from build123d import *

# Parameters (mm, degrees)
F0_R     = 4
F0_R_2   = 22.606
F1_DEPTH = 18


with BuildPart() as f1:
    # F0 (on Front) → F1 (new body)
    with BuildSketch(Plane.XZ):
        with BuildLine():
            ThreePointArc((138.72574, -5.657885), (138.812234, -2.82953), (138.841069, 0))
            ThreePointArc((138.841069, 0), (138.546757, 9.035416), (137.665067, 18.032525))
            ThreePointArc((137.665067, 18.032525), (136.023008, 27.831344), (133.684401, 37.487643))
            ThreePointArc((133.684401, 37.487643), (129.994558, 48.76738), (125.354902, 59.690796))
            ThreePointArc((125.354902, 59.690796), (120.76521, 68.502602), (115.557102, 76.963619))
            ThreePointArc((115.557102, 76.963619), (108.562222, 86.551062), (100.774126, 95.506115))
            ThreePointArc((100.774126, 95.506115), (93.686072, 102.468348), (86.118269, 108.90586))
            ThreePointArc((86.118269, 108.90586), (76.50306, 115.862524), (66.328876, 121.972631))
            ThreePointArc((66.328876, 121.972631), (57.436288, 126.403779), (48.249579, 130.187636))
            ThreePointArc((48.249579, 130.187636), (36.955245, 133.832554), (25.390894, 136.499615))
            ThreePointArc((25.390894, 136.499615), (15.56424, 137.965927), (5.657885, 138.72574))
            ThreePointArc((5.657885, 138.72574), (-6.210007, 138.702121), (-18.032525, 137.665067))
            ThreePointArc((-18.032525, 137.665067), (-27.831344, 136.023008), (-37.487643, 133.684401))
            ThreePointArc((-37.487643, 133.684401), (-48.76738, 129.994558), (-59.690796, 125.354902))
            ThreePointArc((-59.690796, 125.354902), (-68.502602, 120.76521), (-76.963619, 115.557102))
            ThreePointArc((-76.963619, 115.557102), (-86.551062, 108.562222), (-95.506115, 100.774126))
            ThreePointArc((-95.506115, 100.774126), (-102.468348, 93.686072), (-108.90586, 86.118269))
            ThreePointArc((-108.90586, 86.118269), (-115.862524, 76.50306), (-121.972631, 66.328876))
            ThreePointArc((-121.972631, 66.328876), (-126.403779, 57.436288), (-130.187636, 48.249579))
            ThreePointArc((-130.187636, 48.249579), (-133.832554, 36.955245), (-136.499615, 25.390894))
            ThreePointArc((-136.499615, 25.390894), (-137.965927, 15.56424), (-138.72574, 5.657885))
            ThreePointArc((-138.72574, 5.657885), (-138.702121, -6.210007), (-137.665067, -18.032525))
            ThreePointArc((-137.665067, -18.032525), (-136.023008, -27.831344), (-133.684401, -37.487643))
            ThreePointArc((-133.684401, -37.487643), (-129.994558, -48.76738), (-125.354902, -59.690796))
            ThreePointArc((-125.354902, -59.690796), (-120.76521, -68.502602), (-115.557102, -76.963619))
            ThreePointArc((-115.557102, -76.963619), (-108.562222, -86.551062), (-100.774126, -95.506115))
            ThreePointArc((-100.774126, -95.506115), (-93.686072, -102.468348), (-86.118269, -108.90586))
            ThreePointArc((-86.118269, -108.90586), (-76.50306, -115.862524), (-66.328876, -121.972631))
            ThreePointArc((-66.328876, -121.972631), (-57.436288, -126.403779), (-48.249579, -130.187636))
            ThreePointArc((-48.249579, -130.187636), (-36.955245, -133.832554), (-25.390894, -136.499615))
            ThreePointArc((-25.390894, -136.499615), (-15.56424, -137.965927), (-5.657885, -138.72574))
            ThreePointArc((-5.657885, -138.72574), (6.210007, -138.702121), (18.032525, -137.665067))
            ThreePointArc((18.032525, -137.665067), (27.831344, -136.023008), (37.487643, -133.684401))
            ThreePointArc((37.487643, -133.684401), (48.76738, -129.994558), (59.690796, -125.354902))
            ThreePointArc((59.690796, -125.354902), (68.502602, -120.76521), (76.963619, -115.557102))
            ThreePointArc((76.963619, -115.557102), (86.551062, -108.562222), (95.506115, -100.774126))
            ThreePointArc((95.506115, -100.774126), (102.468348, -93.686072), (108.90586, -86.118269))
            ThreePointArc((108.90586, -86.118269), (115.862524, -76.50306), (121.972631, -66.328876))
            ThreePointArc((121.972631, -66.328876), (126.403779, -57.436288), (130.187636, -48.249579))
            ThreePointArc((130.187636, -48.249579), (133.832554, -36.955245), (136.499615, -25.390894))
            ThreePointArc((136.499615, -25.390894), (137.965927, -15.56424), (138.72574, -5.657885))
        make_face()
        with Locations((-86.60254, -50)):
            Circle(F0_R, mode=Mode.SUBTRACT)
        with Locations((0, -35)):
            Circle(F0_R, mode=Mode.SUBTRACT)
        with Locations((86.60254, -50)):
            Circle(F0_R, mode=Mode.SUBTRACT)
        with Locations((-30.310889, 17.5)):
            Circle(F0_R, mode=Mode.SUBTRACT)
        Circle(F0_R_2, mode=Mode.SUBTRACT)
        with Locations((30.310889, 17.5)):
            Circle(F0_R, mode=Mode.SUBTRACT)
        with Locations((0, 100)):
            Circle(F0_R, mode=Mode.SUBTRACT)
        with BuildLine():
            ThreePointArc((-137.665067, -18.032525), (-138.702121, -6.210007), (-138.72574, 5.657885))
            ThreePointArc((-138.72574, 5.657885), (-149.711791, 8.709228), (-159.307768, 14.867253))
            ThreePointArc((-159.307768, 14.867253), (-151.088132, -3.294142), (-137.665067, -18.032525))
        make_face()
        with BuildLine():
            ThreePointArc((-136.499615, 25.390894), (-133.832554, 36.955245), (-130.187636, 48.249579))
            ThreePointArc((-130.187636, 48.249579), (-139.693075, 54.546456), (-146.916457, 63.368405))
            ThreePointArc((-146.916457, 63.368405), (-144.711299, 43.555885), (-136.499615, 25.390894))
        make_face()
        with BuildLine():
            ThreePointArc((-121.972631, 66.328876), (-115.862524, 76.50306), (-108.90586, 86.118269))
            ThreePointArc((-108.90586, 86.118269), (-116.000227, 95.044297), (-120.14394, 105.666616))
            ThreePointArc((-120.14394, 105.666616), (-124.169115, 86.142359), (-121.972631, 66.328876))
        make_face()
        with BuildLine():
            ThreePointArc((-95.506115, 100.774126), (-86.551062, 108.562222), (-76.963619, 115.557102))
            ThreePointArc((-76.963619, 115.557102), (-80.952469, 126.238539), (-81.610896, 137.621443))
            ThreePointArc((-81.610896, 137.621443), (-91.472393, 120.296619), (-95.506115, 100.774126))
        make_face()
        with BuildLine():
            ThreePointArc((-59.690796, 125.354902), (-48.76738, 129.994558), (-37.487643, 133.684401))
            ThreePointArc((-37.487643, 133.684401), (-37.980519, 145.075674), (-35.08921, 156.104924))
            ThreePointArc((-35.08921, 156.104924), (-49.821716, 142.675407), (-59.690796, 125.354902))
        make_face()
        with BuildLine():
            ThreePointArc((-18.032525, 137.665067), (-6.210007, 138.702121), (5.657885, 138.72574))
            ThreePointArc((5.657885, 138.72574), (8.709228, 149.711791), (14.867253, 159.307768))
            ThreePointArc((14.867253, 159.307768), (-3.294142, 151.088132), (-18.032525, 137.665067))
        make_face()
        with BuildLine():
            ThreePointArc((25.390894, 136.499615), (36.955245, 133.832554), (48.249579, 130.187636))
            ThreePointArc((48.249579, 130.187636), (54.546456, 139.693075), (63.368405, 146.916457))
            ThreePointArc((63.368405, 146.916457), (43.555885, 144.711299), (25.390894, 136.499615))
        make_face()
        with BuildLine():
            ThreePointArc((66.328876, 121.972631), (76.50306, 115.862524), (86.118269, 108.90586))
            ThreePointArc((86.118269, 108.90586), (95.044297, 116.000227), (105.666616, 120.14394))
            ThreePointArc((105.666616, 120.14394), (86.142359, 124.169115), (66.328876, 121.972631))
        make_face()
        with BuildLine():
            ThreePointArc((100.774126, 95.506115), (108.562222, 86.551062), (115.557102, 76.963619))
            ThreePointArc((115.557102, 76.963619), (126.238539, 80.952469), (137.621443, 81.610896))
            ThreePointArc((137.621443, 81.610896), (120.296619, 91.472393), (100.774126, 95.506115))
        make_face()
        with BuildLine():
            ThreePointArc((125.354902, 59.690796), (129.994558, 48.76738), (133.684401, 37.487643))
            ThreePointArc((133.684401, 37.487643), (145.075674, 37.980519), (156.104924, 35.08921))
            ThreePointArc((156.104924, 35.08921), (142.675407, 49.821716), (125.354902, 59.690796))
        make_face()
        with BuildLine():
            ThreePointArc((137.665067, 18.032525), (138.546757, 9.035416), (138.841069, 0))
            ThreePointArc((138.841069, 0), (138.812234, -2.82953), (138.72574, -5.657885))
            ThreePointArc((138.72574, -5.657885), (149.711791, -8.709228), (159.307768, -14.867253))
            ThreePointArc((159.307768, -14.867253), (151.088132, 3.294142), (137.665067, 18.032525))
        make_face()
        with BuildLine():
            ThreePointArc((146.916457, -63.368405), (144.711299, -43.555885), (136.499615, -25.390894))
            ThreePointArc((136.499615, -25.390894), (133.832554, -36.955245), (130.187636, -48.249579))
            ThreePointArc((130.187636, -48.249579), (139.693075, -54.546456), (146.916457, -63.368405))
        make_face()
        with BuildLine():
            ThreePointArc((120.14394, -105.666616), (124.169115, -86.142359), (121.972631, -66.328876))
            ThreePointArc((121.972631, -66.328876), (115.862524, -76.50306), (108.90586, -86.118269))
            ThreePointArc((108.90586, -86.118269), (116.000227, -95.044297), (120.14394, -105.666616))
        make_face()
        with BuildLine():
            ThreePointArc((81.610896, -137.621443), (91.472393, -120.296619), (95.506115, -100.774126))
            ThreePointArc((95.506115, -100.774126), (86.551062, -108.562222), (76.963619, -115.557102))
            ThreePointArc((76.963619, -115.557102), (80.952469, -126.238539), (81.610896, -137.621443))
        make_face()
        with BuildLine():
            ThreePointArc((35.08921, -156.104924), (49.821716, -142.675407), (59.690796, -125.354902))
            ThreePointArc((59.690796, -125.354902), (48.76738, -129.994558), (37.487643, -133.684401))
            ThreePointArc((37.487643, -133.684401), (37.980519, -145.075674), (35.08921, -156.104924))
        make_face()
        with BuildLine():
            ThreePointArc((-14.867253, -159.307768), (3.294142, -151.088132), (18.032525, -137.665067))
            ThreePointArc((18.032525, -137.665067), (6.210007, -138.702121), (-5.657885, -138.72574))
            ThreePointArc((-5.657885, -138.72574), (-8.709228, -149.711791), (-14.867253, -159.307768))
        make_face()
        with BuildLine():
            ThreePointArc((-63.368405, -146.916457), (-43.555885, -144.711299), (-25.390894, -136.499615))
            ThreePointArc((-25.390894, -136.499615), (-36.955245, -133.832554), (-48.249579, -130.187636))
            ThreePointArc((-48.249579, -130.187636), (-54.546456, -139.693075), (-63.368405, -146.916457))
        make_face()
        with BuildLine():
            ThreePointArc((-105.666616, -120.14394), (-86.142359, -124.169115), (-66.328876, -121.972631))
            ThreePointArc((-66.328876, -121.972631), (-76.50306, -115.862524), (-86.118269, -108.90586))
            ThreePointArc((-86.118269, -108.90586), (-95.044297, -116.000227), (-105.666616, -120.14394))
        make_face()
        with BuildLine():
            ThreePointArc((-137.621443, -81.610896), (-120.296619, -91.472393), (-100.774126, -95.506115))
            ThreePointArc((-100.774126, -95.506115), (-108.562222, -86.551062), (-115.557102, -76.963619))
            ThreePointArc((-115.557102, -76.963619), (-126.238539, -80.952469), (-137.621443, -81.610896))
        make_face()
        with BuildLine():
            ThreePointArc((-156.104924, -35.08921), (-142.675407, -49.821716), (-125.354902, -59.690796))
            ThreePointArc((-125.354902, -59.690796), (-129.994558, -48.76738), (-133.684401, -37.487643))
            ThreePointArc((-133.684401, -37.487643), (-145.075674, -37.980519), (-156.104924, -35.08921))
        make_face()
    extrude(amount=F1_DEPTH)


solid = f1.part
Could you check a few things on this model? Use its own coordinates, in mm. A direction names the side the tool comes from. Give positions to 0.01 mm unless a question says otherwise; leave off trailing zeros. Write each loop counter-clockwise with the first axis right and the second up, starting at its lowest first coordinate (ties: lowest second). Pieces come first, ordered by that corner, then holes. Notation, with made-up numbers: (80, 17.25) -> (88, 17.25) arc R22 ccw to (88, 51.25) -> close; hole circle Ø10 at (33.5, -10.5). An arc over 180 degrees is marked (long way). Answer as CSV lines item,"result". Start each with the question number.
(1) If we mould it in two halves opening along X, with no side actions, what happens to faces 1 (the face through (-15.7, -8.87, -137.95)), 2 (the face through (-120.834, -8.874, -68.382)), 3 (the face through (49.65, -8.87, -142.89)), 4 (the face through (120.834, -8.874, 68.382))? For each: +X half, -X half, draft (parallel to the pull), parting line (faces both ways), or undercut.
(2) Which directions (+Z, -Z, +X, -X, +Y, -Y) give clear straight access to the entire face, cutting with the end or side of a thin tool? Please do faces 5 (the face through (-93.789, -8.874, -102.374)), 6 (the face through (68.382, -8.874, -120.834)), 7 (the face through (-102.374, -8.874, 93.789)), 8 (the face through (144.785, -8.874, -43.826)), 9 (the face through (90.3, -8.87, -51.53)).
(3) If we section it at C-C, the plane z = -91.5: Write out the boundary of the cut face in (x, y).
(4) I'm going to push flat-ended pins straight in: pin 1 Ø4 at (x, y) = (6.5, -12.5) entering from +Z; pin 2 Ø4 at (y, z) = (-12, -45.5) entering from +X; pin 3 Ø3 at (y, z) = (-13, 8.5) entering from -X. Where does each tip first touch, or does it pass through?
(5) If we section it at A-A, the plane x = 0: Write out the boundary of the cut face in (y, z).
(6) If we section it at B-B, the plane y = -11: Give the number of separate pieces and of enclosed holes in the cut face, and give its area (3 significant figures).
(7) Please list where these lines run through material, in increasing order: line 1 (Z direction, x = -2, y = -4.5); line 2 (Z direction, x = -140, y = -6.5); line 3 (X direction, y = -2.75, z = -47).
Answer list:
1,face 1,"undercut"
1,face 2,"-X half"
1,face 3,"undercut"
1,face 4,"+X half"
2,face 5,"-X, +Y, -Y"
2,face 6,"-Z, +Y, -Y"
2,face 7,"+Z, +Y, -Y"
2,face 8,"+X, +Y, -Y"
2,face 9,"+Y, -Y"
3,outline,"(-120.22, -18) -> (104.43, -18) -> (104.43, 0) -> (-120.22, 0) -> close; (113.69, -18) -> (123.69, -18) -> (123.69, 0) -> (113.69, 0) -> close"
4,pin 1,"z = 157.19"
4,pin 2,"x = 145.66"
4,pin 3,"x = -157.76"
5,outline,"(-18, -153.11) -> (0, -153.11) -> (0, -39) -> (-18, -39) -> close; (-18, -31) -> (0, -31) -> (0, -22.61) -> (-18, -22.61) -> close; (-18, 22.61) -> (0, 22.61) -> (0, 96) -> (-18, 96) -> close; (-18, 104) -> (0, 104) -> (0, 153.11) -> (-18, 153.11) -> close"
6,separate pieces,"1"
6,enclosed holes,"7"
6,area,"64,400 mm^2"
7,line 1,"-154.22 to -38.46, -31.54 to -22.52, 22.52 to 96.54, 103.46 to 151.92"
7,line 2,"-51.85 to -38.18, -16.07 to 5.83, 31.41 to 54.83"
7,line 3,"-145.97 to -89.25, -83.96 to 83.96, 89.25 to 145.55"
